Autodesk Fusion 360 part; units mm, degrees
sketch "Sketch1" plane through (0, 0, 0) normal (0, 0, 1) x (1, 0, 0)
  line L0 (2.72, 5) -> (-2.72, 5)
  line L1 (-5, 2.72) -> (-5, -2.72)
  line L2 (-2.72, -5) -> (2.72, -5)
  line L3 (5, -2.72) -> (5, 2.72)
  line L4 (5, 5) -> (-5, -5) construction
  line L5 (-5, 5) -> (5, -5) construction
  arc A0 (5, 2.72) -> (2.72, 5) centre (2.72, 2.72) ccw
  arc A1 (2.72, -5) -> (5, -2.72) centre (2.72, -2.72) ccw
  arc A2 (-5, -2.72) -> (-2.72, -5) centre (-2.72, -2.72) ccw
  arc A3 (-2.72, 5) -> (-5, 2.72) centre (-2.72, 2.72) ccw
  line L6 (-2.72, -5.2) -> (2.72, -5.2)
  arc A4 (2.72, -5.2) -> (5.2, -2.72) centre (2.72, -2.72) ccw
  line L7 (5.2, -2.72) -> (5.2, 2.72)
  arc A5 (5.2, 2.72) -> (2.72, 5.2) centre (2.72, 2.72) ccw
  line L8 (2.72, 5.2) -> (-2.72, 5.2)
  arc A6 (-2.72, 5.2) -> (-5.2, 2.72) centre (-2.72, 2.72) ccw
  line L9 (-5.2, 2.72) -> (-5.2, -2.72)
  arc A7 (-5.2, -2.72) -> (-2.72, -5.2) centre (-2.72, -2.72) ccw
  line L10 (-2.72, -5.8) -> (2.72, -5.8)
  arc A8 (2.72, -5.8) -> (5.8, -2.72) centre (2.72, -2.72) ccw
  line L11 (5.8, -2.72) -> (5.8, 2.72)
  arc A9 (5.8, 2.72) -> (2.72, 5.8) centre (2.72, 2.72) ccw
  line L12 (2.72, 5.8) -> (-2.72, 5.8)
  arc A10 (-2.72, 5.8) -> (-5.8, 2.72) centre (-2.72, 2.72) ccw
  line L13 (-5.8, 2.72) -> (-5.8, -2.72)
  arc A11 (-5.8, -2.72) -> (-2.72, -5.8) centre (-2.72, -2.72) ccw
  dimension "d1" = 10
  dimension "d2" = 10
  dimension "d3" = 2.28
  dimension "d4" = 0.2
  dimension "d5" = 0.8
extrude "Extrude1" add sketch "Sketch1" along normal blind 3 contours L10 A8 L11 A9 L12 A10 L13 A11
extrude "Extrude2" add sketch "Sketch1" against normal blind 0.5 contours L0 L1 L2 L3 A0 A1 A2 A3 | L6 A4 L7 A5 L8 A6 L9 A7 | L10 A8 L11 A9 L12 A10 L13 A11
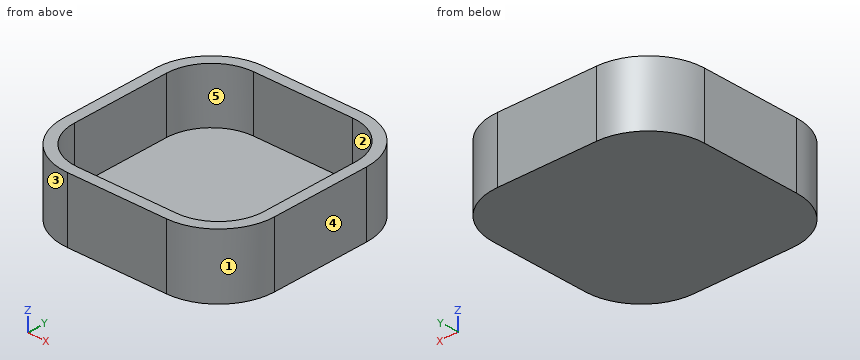
Geometry: final body of the model. Coordinates: model frame, mm. Face numbers are marked on the shaded views. A direction names the side the tool comes from. Coordinates: 2 decimals unless noted, no trailing zeros. Order: outer loops, then holes, each group sorted by start corner. A loop starts at its lowest first (then second) coordinate and runs counter-clockwise, first axis right, second up. Notation, with made-up numbers: (-16, 49.5) - (-10, 49.5) arc R31 cw to (-10, 85.5) - close; hole circle Ø4 at (63, -12). An arc over 180 degrees is marked (long way). Write each question's results on one line, items separated by ' | '.
(1) Section query B-B, the plane x = -0.5. Return the cut outline in (y, z).
Values found:
outline: (-5.8, -0.5) - (5.8, -0.5) - (5.8, 3) - (5.2, 3) - (5.2, 0) - (-5.2, 0) - (-5.2, 3) - (-5.8, 3) - close
(2) Mould query, pull axis X, two halves, no side actions, for the marked faces 3, 4 and 5. Classes: +X half, -X half, draft (parallel to the pull), parting line (faces both ways), or undercut.
Values found:
face 3: -X half | face 4: +X half | face 5: undercut
(3) Set-up query: the marked faces 1 and 2. Return all of +Z, -Z, +X, -X, +Y, -Y with unobstructed straight access to the full face (end or side cutting, diameter ignored); none if empty.
Values found:
face 1: +Z, -Z, +X, -Y | face 2: +Z
(4) Line query: line 1 (Y direction, x = -2.25, z = 1); line 2 (Z direction, x = 4.75, y = 3.25). Output: solid intervals per line, ascending. Write a range as [from, to].
Values found:
line 1: y = [-5.8, -5.2], [5.2, 5.8] | line 2: z = [-0.5, 0]
(5) First-contact query: pin 1 Ø3 at (x, y) = (-1.5, 1.5) entering from +Z. Flat tip, straight axial feed; report the tip coordinate or a pass-through.
Values found:
pin 1: stops at z = 0
(6) Section query A-A, the plane z = 0.3. Return the cut outline in (x, y).
Values found:
outline: (-5.8, -2.72) arc R3.08 ccw to (-2.72, -5.8) - (2.72, -5.8) arc R3.08 ccw to (5.8, -2.72) - (5.8, 2.72) arc R3.08 ccw to (2.72, 5.8) - (-2.72, 5.8) arc R3.08 ccw to (-5.8, 2.72) - close; hole (-5.2, -2.72) arc R2.48 ccw to (-2.72, -5.2) - (2.72, -5.2) arc R2.48 ccw to (5.2, -2.72) - (5.2, 2.72) arc R2.48 ccw to (2.72, 5.2) - (-2.72, 5.2) arc R2.48 ccw to (-5.2, 2.72) - close
